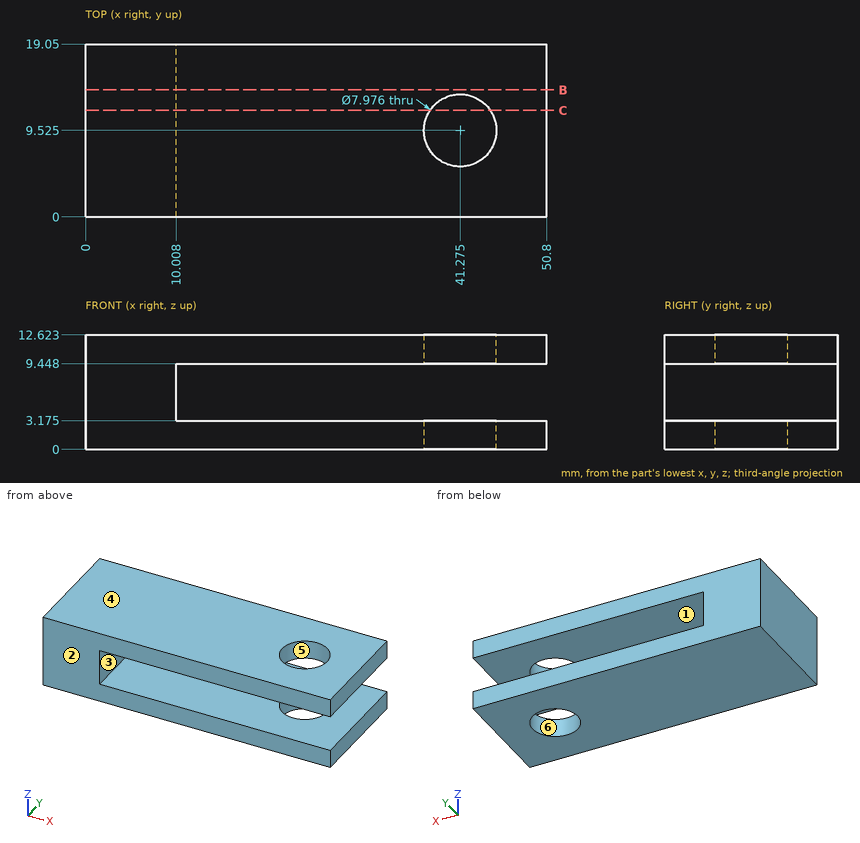
Job drawing, mm, ordinate dimensions from the low corner. One solid piece. A direction names the side the tool comes from. Give positions to 0.01 mm unless a question says otherwise; leave off trailing zeros. Write each loop counter-clockwise with the first axis right and the second up, starting at its lowest first coordinate (ties: lowest second). Pieces come first, ordered by that corner, then holes. Notation, with made-up numbers: M 34,55.25 L 49,55.25 A14 cw 49,78.25 Z; hole C -36.75,58.25 d9. An arc over 180 degrees is marked long. One line per item, written item: value. Start each with the question number.
Q1. Saw through at C-C, the plane y = 11.75. Write the cut outline in (x, z) (1 decimal), plus the area to 3 significant figures.
Q2. Two-plate mould, pull along X, no slides. Class the marked faces 3, 4, 5 and 6: +X half, -X half, draft (parallel to the pull), parting line (faces both ways), or undercut.
Q3. Saw through at B-B, the plane y = 14. Write the cut outline in (x, z) (1 decimal).
Q4. 3-axis set-ups, long thin cutter, end or side, ignore diameter. For the marked faces 1 and 2: which of +Z, -Z, +X, -X, +Y, -Y reach the whole face in a straight line?
Q5. Probe probe 1 along Z at (x, y) = (28.5, 13.5) (1 decimal); probe 2 along X at (y, z) = (10.5, 0.5); probe 3 along X at (y, z) = (14, 6.5). List the from-to ranges inside material, lowest first. Write a range as [from, to].
Output values:
1. outline: M 0,0 L 38,0 L 38,3.2 L 10,3.2 L 10,9.4 L 38,9.4 L 38,12.6 L 0,12.6 Z; M 44.6,0 L 50.8,0 L 50.8,3.2 L 44.6,3.2 Z; M 44.6,9.4 L 50.8,9.4 L 50.8,12.6 L 44.6,12.6 Z
1. area: 343 mm²
2. face 3: +X half
2. face 4: draft
2. face 5: undercut
2. face 6: undercut
3. outline: M 0,0 L 50.8,0 L 50.8,3.2 L 10,3.2 L 10,9.4 L 50.8,9.4 L 50.8,12.6 L 0,12.6 Z
4. face 1: +X, +Y, -Y
4. face 2: +Z, -Z, +X, -X, -Y
5. probe 1: z = [0, 3.2], [9.4, 12.6]
5. probe 2: x = [0, 37.41], [45.14, 50.8]
5. probe 3: x = [0, 10.01]
